Geometry: final body of the model. Coordinates: model frame, mm. Give positions to 0.01 mm unless a question says otherwise; leave off trailing zeros. Loops run counter-clockwise (first coordinate to the right, second up) from the corner with the lowest first, then second, coordinate; pieces in that order, holes last. Notation, with made-up numbers: (67.5, 26.25) - (80.5, 26.25) arc R20 cw to (80.5, 54.25) - close; hole circle Ø4 at (73, -23.5). An arc over 180 degrees is marked (long way). Use CSV: the item, a comma, the result in double quotes. Start each with the question number.
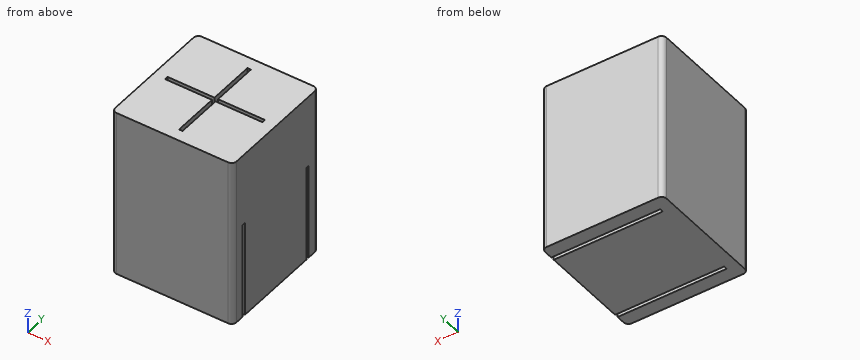
```python
from build123d import *

# Parameters (mm, degrees)
SKETCH1_W           = 63.5
SKETCH1_H           = 63.5
BOSS_EXTRUDE1_DEPTH = 25.4
SKETCH1_7_W         = 63.5
SKETCH1_7_H         = 63.5
BOSS_EXTRUDE2_DEPTH = 63.5
CUT_EXTRUDE1_START  = -6.35
SKETCH2_W           = 50.8
SKETCH2_H           = 1.8415
CUT_EXTRUDE1_DEPTH  = 89.9
FILLET1_R           = 2.54


with BuildPart() as part:
    # Sketch1 → Boss-Extrude1 (new body)
    with BuildSketch(Plane.XY):
        Rectangle(SKETCH1_W, SKETCH1_H)
        Polygon((-0.92075, -0.92075), (-25.527, -0.92075), (-25.527, 0.92075), (-0.92075, 0.92075), (-0.92075, 25.527), (0.92075, 25.527), (0.92075, 0.92075), (25.527, 0.92075), (25.527, -0.92075), (0.92075, -0.92075), (0.92075, -25.527), (-0.92075, -25.527), align=None, mode=Mode.SUBTRACT)
    extrude(amount=BOSS_EXTRUDE1_DEPTH)

    # Sketch1_7 → Boss-Extrude2 (add)
    with BuildSketch(Plane.XY):
        Rectangle(SKETCH1_7_W, SKETCH1_7_H)
    extrude(amount=-BOSS_EXTRUDE2_DEPTH)

    # Sketch2 → Cut-Extrude1 (cut, through all)
    with BuildSketch(Plane.ZY.offset(31.75).offset(CUT_EXTRUDE1_START)):
        with Locations((-38.1, 23.8125)):
            Rectangle(SKETCH2_W, SKETCH2_H)
        with Locations((-38.1, -23.8125)):
            Rectangle(SKETCH2_W, SKETCH2_H)
    extrude(amount=-CUT_EXTRUDE1_DEPTH, mode=Mode.SUBTRACT)

    # Fillet1
    fillet1_edges = [part.edges().sort_by_distance(p)[0] for p in [
        (-31.75, -31.75, -19.05),
        (-31.75, 31.75, -19.05),
        (31.75, 31.75, -19.05),
        (31.75, -31.75, -19.05),
    ]]
    fillet(fillet1_edges, radius=FILLET1_R)


solid = part.part
```
Item 1: Section A-A (z = 16). Output: boundary loops of the cut face in (x, y), plus the area to 3 significant figures.
Item 2: Ray query, probe 1 along Y at (x, z) = (-23.5, -46); probe 2 along X at (y, z) = (3.5, 7). Return the intervals inside material, ascending.
Item 3: Section D-D (x = -23). Output: boundary loops of the cut face in (y, z).
Item 4: Pin query (flat end, axial travel): pin 1 Ø0.9 at (x, y) = (12, 24) entering from -Z; pin 2 Ø2 at (x, y) = (5.5, -24) entering from -Z. Return the tip coordinate at first contact, or that it passes through.
Item 5: Section B-B (x = 27.5). Output: boundary loops of the cut face in (y, z), plus the area to 3 significant figures.
Item 6: Section C-C (z = -47). Output: boundary loops of the cut face in (x, y).
Outcome:
1,outline,"(-31.75, -29.21) arc R2.54 ccw to (-29.21, -31.75) - (29.21, -31.75) arc R2.54 ccw to (31.75, -29.21) - (31.75, 29.21) arc R2.54 ccw to (29.21, 31.75) - (-29.21, 31.75) arc R2.54 ccw to (-31.75, 29.21) - close; hole (-25.53, -0.92) - (-0.92, -0.92) - (-0.92, -25.53) - (0.92, -25.53) - (0.92, -0.92) - (25.53, -0.92) - (25.53, 0.92) - (0.92, 0.92) - (0.92, 25.53) - (-0.92, 25.53) - (-0.92, 0.92) - (-25.53, 0.92) - close"
1,area,"3,840 mm2"
2,probe 1,"y = -31.75 to -24.73, -22.89 to 22.89, 24.73 to 31.75"
2,probe 2,"x = -31.75 to -0.92, 0.92 to 31.75"
3,outline,"(-31.75, -63.5) - (-24.73, -63.5) - (-24.73, -12.7) - (-22.89, -12.7) - (-22.89, -63.5) - (22.89, -63.5) - (22.89, -12.7) - (24.73, -12.7) - (24.73, -63.5) - (31.75, -63.5) - (31.75, 25.4) - (0.92, 25.4) - (0.92, 0) - (-0.92, 0) - (-0.92, 25.4) - (-31.75, 25.4) - close"
4,pin 1,"stops at z = -12.7"
4,pin 2,"stops at z = -63.5"
5,outline,"(-31.75, -63.5) - (-24.73, -63.5) - (-24.73, -12.7) - (-22.89, -12.7) - (-22.89, -63.5) - (22.89, -63.5) - (22.89, -12.7) - (24.73, -12.7) - (24.73, -63.5) - (31.75, -63.5) - (31.75, 25.4) - (-31.75, 25.4) - close"
5,area,"5,460 mm2"
6,outline,"(-31.75, -29.21) arc R2.54 ccw to (-29.21, -31.75) - (29.21, -31.75) arc R2.54 ccw to (31.75, -29.21) - (31.75, -24.73) - (-25.4, -24.73) - (-25.4, -22.89) - (31.75, -22.89) - (31.75, 22.89) - (-25.4, 22.89) - (-25.4, 24.73) - (31.75, 24.73) - (31.75, 29.21) arc R2.54 ccw to (29.21, 31.75) - (-29.21, 31.75) arc R2.54 ccw to (-31.75, 29.21) - close"
